```python
from build123d import *

# Parameters (mm, degrees)
SKETCH1_W            = 180
SKETCH1_H            = 65
SKETCH1_W_2          = 171.45
SKETCH1_H_2          = 57.15
BOSS_EXTRUDE1_DEPTH  = 10
SKETCH2_W            = 180
SKETCH2_H            = 65
BOSS_EXTRUDE2_DEPTH  = 2.5
SKETCH3_W            = 19.05
SKETCH3_H            = 4.647704017
SKETCH3_H_2          = 3.172295983
BOSS_EXTRUDE3_DEPTH  = 2.5
SKETCH4_W            = 2.440634246
SKETCH4_H            = 20.32
BOSS_EXTRUDE4_DEPTH  = 19.05
SKETCH5_W            = 19.05
SKETCH5_H            = 25.298590684
BOSS_EXTRUDE5_DEPTH  = 2.5
BOSS_EXTRUDE6_DEPTH  = 19.05
SKETCH7_W            = 35
SKETCH7_H            = 5.223578232
BOSS_EXTRUDE7_DEPTH  = 4
SKETCH8_W            = 1.900028328
SKETCH8_H            = 5.223578232
SKETCH8_W_2          = 1.933775308
BOSS_EXTRUDE8_DEPTH  = 35
SKETCH9_W            = 25.32
SKETCH9_H            = 2.501981816
BOSS_EXTRUDE9_DEPTH  = 19.05
SKETCH10_W           = 20.346164675
SKETCH10_H           = 20.35236298
SKETCH10_W_2         = 20.379365754
SKETCH10_H_2         = 20.32
BOSS_EXTRUDE10_DEPTH = 19.05
SKETCH11_W           = 21.053847509
SKETCH11_H           = 26.24333769
SKETCH11_W_2         = 20.65238494
SKETCH11_H_2         = 27.151183987
CUT_EXTRUDE1_DEPTH   = 219.146485719
SKETCH12_W           = 32.74513921
SKETCH12_H           = 12.5
BOSS_EXTRUDE11_DEPTH = 10
SKETCH13_R           = 2.5
BOSS_EXTRUDE12_DEPTH = 50
BOSS_EXTRUDE13_START = -25
BOSS_EXTRUDE13_DEPTH = 25
BOSS_EXTRUDE14_DEPTH = 2.5
BOSS_EXTRUDE15_DEPTH = 2.5


with BuildPart() as part:
    # Sketch1 → Boss-Extrude1 (new body)
    with BuildSketch(Plane(origin=(0, 0, 0), x_dir=(1, 0, 0), z_dir=(0, 1, 0))):
        with Locations((85.674229947, 28.51722294)):
            Rectangle(SKETCH1_W, SKETCH1_H)
        with Locations((85.725, 28.575)):
            Rectangle(SKETCH1_W_2, SKETCH1_H_2, mode=Mode.SUBTRACT)
    extrude(amount=BOSS_EXTRUDE1_DEPTH)

    # Sketch2 → Boss-Extrude2 (add)
    with BuildSketch(Plane(origin=(0, 0, 0), x_dir=(-1, 0, 0), z_dir=(0, -1, 0))):
        with Locations((-85.674229947, 28.51722294)):
            Rectangle(SKETCH2_W, SKETCH2_H)
    extrude(amount=BOSS_EXTRUDE2_DEPTH)

    # Sketch3 → Boss-Extrude3 (add)
    with BuildSketch(Plane(origin=(175.674229947, 0, 0), x_dir=(0, 0, -1), z_dir=(1, 0, 0))):
        with Locations((38.04222294, 12.323852009)):
            Rectangle(SKETCH3_W, SKETCH3_H)
        Polygon((28.51722294, 10), (28.51722294, 3.75), (28.51722294, -2.5), (47.56722294, -2.5), (47.56722294, 10), align=None)
        with Locations((38.04222294, -4.086147992)):
            Rectangle(SKETCH3_W, SKETCH3_H_2)
    extrude(amount=BOSS_EXTRUDE3_DEPTH)

    # Sketch4 → Boss-Extrude4 (add)
    with BuildSketch(Plane(origin=(0, 0, -47.56722294), x_dir=(-1, 0, 0), z_dir=(0, 0, -1))):
        Polygon((-200.994229947, 17.126484518), (-200.994229947, 14.647704017), (-198.553595701, 14.647704017), (-178.174229947, 14.647704017), (-175.674229947, 14.647704017), (-175.674229947, 17.126484518), align=None)
        with Locations((-199.773912824, 4.487704017)):
            Rectangle(SKETCH4_W, SKETCH4_H)
        Polygon((-198.553595701, -5.672295983), (-200.994229947, -5.672295983), (-200.994229947, -8.172106166), (-175.674229947, -8.172106166), (-175.674229947, -5.672295983), (-178.174229947, -5.672295983), align=None)
    extrude(amount=-BOSS_EXTRUDE4_DEPTH)

    # Sketch5 → Boss-Extrude5 (add)
    with BuildSketch(Plane.ZY.offset(4.325770053)):
        with Locations((-38.04222294, 4.477189176)):
            Rectangle(SKETCH5_W, SKETCH5_H)
    extrude(amount=BOSS_EXTRUDE5_DEPTH)

    # Sketch6 → Boss-Extrude6 (add)
    with BuildSketch(Plane.XY.offset(-28.51722294)):
        Polygon((-29.645770053, -8.172106166), (-27.171934728, -8.172106166), (-27.171934728, 14.68223863), (-4.325770053, 14.68223863), (-4.325770053, 17.115716116), (-29.645770053, 17.115716116), align=None)
    extrude(amount=-BOSS_EXTRUDE6_DEPTH)

    # Sketch7 → Boss-Extrude7 (add)
    with BuildSketch(Plane.XY.offset(3.98277706)):
        with Locations((86.801660342, 7.388210884)):
            Rectangle(SKETCH7_W, SKETCH7_H)
        with Locations((86.801660342, 0.111789116)):
            Rectangle(SKETCH7_W, SKETCH7_H)
    extrude(amount=BOSS_EXTRUDE7_DEPTH)

    # Sketch8 → Boss-Extrude8 (add)
    with BuildSketch(Plane.XY.offset(3.98277706)):
        with Locations((70.251674506, 7.388210884)):
            Rectangle(SKETCH8_W, SKETCH8_H)
        with Locations((70.251674506, 0.111789116)):
            Rectangle(SKETCH8_W, SKETCH8_H)
        with Locations((103.334772688, 0.111789116)):
            Rectangle(SKETCH8_W_2, SKETCH8_H)
        with Locations((103.334772688, 7.388210884)):
            Rectangle(SKETCH8_W_2, SKETCH8_H)
    extrude(amount=BOSS_EXTRUDE8_DEPTH)

    # Sketch9 → Boss-Extrude9 (add)
    with BuildSketch(Plane.XY.offset(-28.51722294)):
        with Locations((-16.985770053, -6.921115258)):
            Rectangle(SKETCH9_W, SKETCH9_H)
    extrude(amount=-BOSS_EXTRUDE9_DEPTH)

    # Sketch10 → Boss-Extrude10 (add)
    # profile 1 of 2: a face of its own
    with BuildSketch(Plane.XY.offset(-28.51722294)):
        with BuildLine():
            ThreePointArc((0, 10.117261054), (-34.872965087, 4.477189176), (0, -1.162882702))
            Line((0, -1.162882702), (0, 10.117261054))
        make_face()
        with Locations((-16.998852391, 4.50605714)):
            Rectangle(SKETCH10_W, SKETCH10_H, mode=Mode.SUBTRACT)
    # profile 2 of 2: a face of its own
    with BuildSketch(Plane.XY.offset(-28.51722294)):
        with BuildLine():
            Line((171.45, 10.410405146), (171.45, -1.456026794))
            ThreePointArc((171.45, -1.456026794), (206.230605911, 4.477189176), (171.45, 10.410405146))
        make_face()
        with Locations((188.363912824, 4.487704017)):
            Rectangle(SKETCH10_W_2, SKETCH10_H_2, mode=Mode.SUBTRACT)
    extrude(amount=-BOSS_EXTRUDE10_DEPTH)

    # Sketch11 → Cut-Extrude1 (cut, through all)
    with BuildSketch(Plane.XY.offset(-28.51722294)):
        with BuildLine():
            Line((-53.173508904, 4.50605714), (-34.8729418, 4.50605714))
            ThreePointArc((-34.8729418, 4.50605714), (-33.104696604, 12.232894836), (-28.171934728, 18.437616596))
            Line((-28.171934728, 18.437616596), (-28.171934728, 29.671454137))
            Line((-28.171934728, 29.671454137), (-53.381023661, 29.671454137))
            Line((-53.381023661, 29.671454137), (-53.381023661, 4.50605714))
            Line((-53.381023661, 4.50605714), (-53.173508904, 4.50605714))
        make_face()
        with BuildLine():
            ThreePointArc((-29.645770053, -8.161337764), (-33.520115813, -2.347890017), (-34.8729418, 4.50605714))
            Line((-34.8729418, 4.50605714), (-53.173508904, 4.50605714))
            Line((-53.173508904, 4.50605714), (-53.173508904, -18.45755641))
            Line((-53.173508904, -18.45755641), (-28.171934728, -18.45755641))
            Line((-28.171934728, -18.45755641), (-28.171934728, -9.483238244))
            ThreePointArc((-28.171934728, -9.483238244), (-28.921483903, -8.847768144), (-29.635015336, -8.172106166))
            Line((-29.635015336, -8.172106166), (-29.645770053, -8.172106166))
            Line((-29.645770053, -8.172106166), (-29.645770053, -8.161337764))
        make_face()
        with BuildLine():
            Line((-34.8729418, 4.50605714), (-28.171934728, 4.50605714))
            Line((-28.171934728, 4.50605714), (-28.171934728, 18.437616596))
            ThreePointArc((-28.171934728, 18.437616596), (-33.104696604, 12.232894836), (-34.8729418, 4.50605714))
        make_face()
        with BuildLine():
            Line((-28.171934728, -9.483238244), (-28.171934728, 4.50605714))
            Line((-28.171934728, 4.50605714), (-34.8729418, 4.50605714))
            ThreePointArc((-34.8729418, 4.50605714), (-33.520115813, -2.347890017), (-29.645770053, -8.161337764))
            Line((-29.645770053, -8.161337764), (-29.645770053, -8.172106166))
            Line((-29.645770053, -8.172106166), (-29.635015336, -8.172106166))
            ThreePointArc((-29.635015336, -8.172106166), (-28.921483903, -8.847768144), (-28.171934728, -9.483238244))
        make_face()
        with Locations((210.080519455, 17.609372862)):
            Rectangle(SKETCH11_W, SKETCH11_H)
        with Locations((209.879788171, -9.087887976)):
            Rectangle(SKETCH11_W_2, SKETCH11_H_2)
    extrude(amount=-CUT_EXTRUDE1_DEPTH, mode=Mode.SUBTRACT)

    # Sketch12 → Boss-Extrude11 (add)
    with BuildSketch(Plane(origin=(0, 0, -61.01722294), x_dir=(-1, 0, 0), z_dir=(0, 0, -1))):
        with Locations((-85.674229947, 3.75)):
            Rectangle(SKETCH12_W, SKETCH12_H)
    extrude(amount=BOSS_EXTRUDE11_DEPTH)

    # Sketch13 → Boss-Extrude12 (add)
    with BuildSketch(Plane(origin=(0, 10, 0), x_dir=(1, 0, 0), z_dir=(0, 1, 0))):
        with Locations(Location((85.674229947, 66.01722294, 0), (0, 0, 90))):
            Circle(SKETCH13_R)
    extrude(amount=BOSS_EXTRUDE12_DEPTH)

    # Sketch14 → Boss-Extrude13 (add)
    with BuildSketch(Plane(origin=(0, 60, 0), x_dir=(1, 0, 0), z_dir=(0, 1, 0)).offset(BOSS_EXTRUDE13_START)):
        with BuildLine():
            Line((84.674229947, 68.308510788), (84.674229947, 66.01722294))
            Line((84.674229947, 66.01722294), (86.674229947, 66.01722294))
            Line((86.674229947, 66.01722294), (86.674229947, 68.308510788))
            ThreePointArc((86.674229947, 68.308510788), (85.674229947, 68.51722294), (84.674229947, 68.308510788))
        make_face()
        with BuildLine():
            Line((86.674229947, 66.01722294), (84.674229947, 66.01722294))
            Line((84.674229947, 66.01722294), (84.674229947, 63.725935093))
            ThreePointArc((84.674229947, 63.725935093), (85.674229947, 63.51722294), (86.674229947, 63.725935093))
            Line((86.674229947, 63.725935093), (86.674229947, 66.01722294))
        make_face()
        with BuildLine():
            Line((84.674229947, 96.01722294), (84.674229947, 68.308510788))
            ThreePointArc((84.674229947, 68.308510788), (85.674229947, 68.51722294), (86.674229947, 68.308510788))
            Line((86.674229947, 68.308510788), (86.674229947, 96.01722294))
            Line((86.674229947, 96.01722294), (84.674229947, 96.01722294))
        make_face()
    extrude(amount=BOSS_EXTRUDE13_DEPTH)

    # Sketch15 → Boss-Extrude14 (add)
    with BuildSketch(Plane(origin=(86.674229947, 0, 0), x_dir=(0, 0, -1), z_dir=(1, 0, 0))):
        Polygon((86.590113791, 57.949199479), (74.364516101, 47.274610451), (84.462974004, 47.274610451), (74.205725369, 36.241603515), (91.143359189, 49.065886488), (80.020746684, 49.909078542), align=None)
    extrude(amount=BOSS_EXTRUDE14_DEPTH)

    # Sketch16 → Boss-Extrude15 (add)
    with BuildSketch(Plane.ZY.offset(-84.674229947)):
        Polygon((-88.831415439, 54.480665097), (-88.831415439, 49.480665097), (-83.207775472, 46.244467981), (-83.207775472, 41.244467981), (-88.831415439, 46.244467981), (-88.831415439, 41.244467981), (-83.320105395, 36.799352745), (-77.00848732, 41.244467981), (-77.00848732, 46.244467981), (-83.207775472, 49.480665097), (-83.207775472, 54.480665097), (-77.00848732, 49.480665097), (-77.00848732, 54.480665097), (-83.207775472, 58.956719844), align=None)
    extrude(amount=BOSS_EXTRUDE15_DEPTH)


solid = part.part
```
Can you work these out from the model? Positions are in its coordinate system, mm. A direction names the side the tool comes from. Coordinates: 2 decimals unless noted, no trailing zeros. Order: outer loops, then holes, each group sorted by start corner. A loop starts at its lowest first (then second) coordinate and runs counter-clockwise, first axis right, second up. Notation, with made-up numbers: (3, -23.75) - (55, -23.75) arc R27 ccw to (55, 12.25) - close; hole circle Ø3 at (23.25, 50.5). An arc over 180 degrees is marked (long way). Answer in a Markdown table with one row per item.
1. For faces 1 (the flat face through (171.45, 5, -28)), 2 (the flat face through (-17, 14.682, -38)), 3 (the flat face through (104.302, 0, 21)), which set-ups out of +Z, -Z, +X, -X, +Y, -Y let a thin tool reach every point of the face, with its end or its side?
Reply:
| item | result |
|---|---|
| face 1 | +Y |
| face 2 | +Z, -Z |
| face 3 | +Z, +X, +Y, -Y |
2. Suppose I cut it at C-C (z = -16.5). Please give me the cut outline in (x, y).
Reply:
| item | result |
|---|---|
| outline | (-4.33, -2.5) - (175.67, -2.5) - (175.67, 10) - (171.45, 10) - (171.45, 0) - (0, 0) - (0, 10) - (-4.33, 10) - close |
3. Suppose I cut it at A-A (z = 21). Please give me the cut outline in (x, y).
Reply:
| item | result |
|---|---|
| outline | (69.3, -2.5) - (71.2, -2.5) - (71.2, 2.72) - (69.3, 2.72) - close; (69.3, 4.78) - (71.2, 4.78) - (71.2, 10) - (69.3, 10) - close; (102.37, -2.5) - (104.3, -2.5) - (104.3, 2.72) - (102.37, 2.72) - close; (102.37, 4.78) - (104.3, 4.78) - (104.3, 10) - (102.37, 10) - close |
4. If I drill on line 1 along Z through (x, y) = (28.5, 3); line 2 along Z through (x, y) = (91, -1.5); line 3 along Y through (x, z) = (81.5, -64), over which ranges is the centre line in solid material (lowest first)?
Reply:
| item | result |
|---|---|
| line 1 | z = -61.02 to -57.15, 0 to 3.98 |
| line 2 | z = -71.02 to 7.98 |
| line 3 | y = -2.5 to 10 |
5. Suppose I cut it at B-B (x = 40). Please give me the cut outline in (y, z).
Reply:
| item | result |
|---|---|
| outline | (-2.5, -61.02) - (10, -61.02) - (10, -57.15) - (0, -57.15) - (0, 0) - (10, 0) - (10, 3.98) - (-2.5, 3.98) - close |
6. Suppose I cut it at D-D (z = -39). Please give me the cut outline in (x, y).
Reply:
| item | result |
|---|---|
| outline | (-28.17, -9.48) arc R17.89 ccw to (-0.5, -2.5) - (171.85, -2.5) arc R17.9 ccw to (199.55, -9.47) - (199.55, 18.42) arc R17.9 ccw to (171.45, 10.41) - (171.45, 0) - (0, 0) - (0, 10.12) arc R17.89 ccw to (-28.17, 18.44) - close; hole (-27.17, -5.67) - (-6.83, -5.67) - (-6.83, 14.68) - (-27.17, 14.68) - close; hole (178.17, -5.67) - (198.55, -5.67) - (198.55, 14.65) - (178.17, 14.65) - close |
7. If we mould it in two halves opening along Z, with no side actions, what happens to faces 4 (the flat face through (0, 5, -28)), 5 (the flat face through (-27.172, 4, -38)), 6 (the flat face through (87, 0, -29))? For each: pulls with the +Z half, pulls with the -Z half, needs draft (parallel to the pull), parting line crosses it, or undercut.
Reply:
| item | result |
|---|---|
| face 4 | undercut |
| face 5 | needs draft |
| face 6 | undercut |
8. For pin 1 (8 mm diameter, centred on x = 65, y = 3, fed in from +Z); pin 2 (1.2 mm diameter, centred on x = 83.5, y = 52, fed in from +Z); pin 3 (3 mm diameter, centred on y = 4, z = -70, fed in from +X), each with a flat end and sliding along its axis, tell me the tip position at first contact or that it passes through.
Reply:
| item | result |
|---|---|
| pin 1 | stops at z = 3.98 |
| pin 2 | stops at z = -64.08 |
| pin 3 | stops at x = 102.05 |
